from build123d import *

# Parameters (mm, degrees)
SKETCH1_W           = 150
SKETCH1_H           = 150
BOSS_EXTRUDE1_DEPTH = 2.5
CUT_EXTRUDE1_DEPTH  = 5
SKETCH3_R           = 1.55
CUT_EXTRUDE2_DEPTH  = 5
CUT_EXTRUDE3_DEPTH  = 5


with BuildPart() as part:
    # Sketch1 → Boss-Extrude1 (new body, symmetric)
    with BuildSketch(Plane(origin=(0, 0, 0), x_dir=(1, 0, 0), z_dir=(0, 1, 0))):
        Rectangle(SKETCH1_W, SKETCH1_H)
    extrude(amount=BOSS_EXTRUDE1_DEPTH, both=True)

    # Sketch2 → Cut-Extrude1 (cut)
    with BuildSketch(Plane(origin=(0, 2.5, 0), x_dir=(1, 0, 0), z_dir=(0, 1, 0))):
        Polygon((50.251262658, 75), (75, 75), (75, 50.251262658), align=None)
        Polygon((-75, 75), (-75, 50.251262658), (-50.251262658, 75), align=None)
        Polygon((-50.251262658, -75), (-75, -75), (-75, -50.251262658), align=None)
        Polygon((75, -75), (75, -50.251262658), (50.251262658, -75), align=None)
    extrude(amount=-CUT_EXTRUDE1_DEPTH, mode=Mode.SUBTRACT)

    # Sketch3 → Cut-Extrude2 (cut)
    with BuildSketch(Plane(origin=(0, 2.5, 0), x_dir=(1, 0, 0), z_dir=(0, 1, 0))):
        with Locations((69.343145751, 50.251262658)):
            Circle(SKETCH3_R)
        with Locations((53.786796564, 34.694913472)):
            Circle(SKETCH3_R)
        with Locations((34.694913472, 53.786796564)):
            Circle(SKETCH3_R)
        with Locations((50.251262658, 69.343145751)):
            Circle(SKETCH3_R)
        with Locations((-69.343145751, 50.251262658)):
            Circle(SKETCH3_R)
        with Locations((-53.786796564, 34.694913472)):
            Circle(SKETCH3_R)
        with Locations((-34.694913472, 53.786796564)):
            Circle(SKETCH3_R)
        with Locations((-50.251262658, 69.343145751)):
            Circle(SKETCH3_R)
        with Locations((-53.786796564, -34.694913472)):
            Circle(SKETCH3_R)
        with Locations((-69.343145751, -50.251262658)):
            Circle(SKETCH3_R)
        with Locations((-34.694913472, -53.786796564)):
            Circle(SKETCH3_R)
        with Locations((-50.251262658, -69.343145751)):
            Circle(SKETCH3_R)
        with Locations((69.343145751, -50.251262658)):
            Circle(SKETCH3_R)
        with Locations((53.786796564, -34.694913472)):
            Circle(SKETCH3_R)
        with Locations((34.694913472, -53.786796564)):
            Circle(SKETCH3_R)
        with Locations((50.251262658, -69.343145751)):
            Circle(SKETCH3_R)
    extrude(amount=-CUT_EXTRUDE2_DEPTH, mode=Mode.SUBTRACT)

    # Sketch4 → Cut-Extrude3 (cut)
    with BuildSketch(Plane(origin=(0, 2.5, 0), x_dir=(1, 0, 0), z_dir=(0, 1, 0))):
        with BuildLine():
            Line((24, 26), (54, 26))
            ThreePointArc((54, 26), (55, 25), (54, 24))
            Line((54, 24), (24, 24))
            ThreePointArc((24, 24), (23, 25), (24, 26))
        make_face()
        with BuildLine():
            Line((24, -26), (54, -26))
            ThreePointArc((54, -26), (55, -25), (54, -24))
            Line((54, -24), (24, -24))
            ThreePointArc((24, -24), (23, -25), (24, -26))
        make_face()
        with BuildLine():
            Line((-24, -26), (-54, -26))
            ThreePointArc((-54, -26), (-55, -25), (-54, -24))
            Line((-54, -24), (-24, -24))
            ThreePointArc((-24, -24), (-23, -25), (-24, -26))
        make_face()
        with BuildLine():
            Line((-24, 26), (-54, 26))
            ThreePointArc((-54, 26), (-55, 25), (-54, 24))
            Line((-54, 24), (-24, 24))
            ThreePointArc((-24, 24), (-23, 25), (-24, 26))
        make_face()
    extrude(amount=-CUT_EXTRUDE3_DEPTH, mode=Mode.SUBTRACT)


solid = part.part
Verification items for the finished model (mm, model axes). A direction names the side the tool comes from. Give positions to 0.01 mm unless a question says otherwise; leave off trailing zeros. Order: outer loops, then holes, each group sorted by start corner. A loop starts at its lowest first (then second) coordinate and runs counter-clockwise, first axis right, second up. Notation, with made-up numbers: M 53,19 L 89,19 A23 cw 89,52 Z; hole C 5,50.5 d9. An arc over 180 degrees is marked long. Answer as a JSON object with one key per item and string values. Group by question number.
1) Mould release check, pull along X, two halves, no side actions. Record for faces 1 (the face through (-1, 2.5, -1)), 2 (the face through (39, 0, 24)), 3 (the face through (62.8, 0.04, 62.45)): released by +X, released by -X, zero draft, split by the parting line, or undercut.
2) Cross-section at A-A (x = 40.5). Enter the section's corners in (y, z).
3) Depth check by flat-ended pin: pin 1 Ø1.9 at (x, z) = (-34.69, -53.79) entering from +Y; pin 2 Ø1.5 at (x, y) = (-56.5, 1) entering from +Z. Enter the tip coordinate at first touch or a pass-through.
4) Scan lines: line 1 along Z through (x, y) = (26.5, -1.1); line 2 along Z through (x, y) = (51, 1.25); line 3 along X through (y, z) = (1.35, -53). Record each from-to range of solid material in increasing order. Write a range as [from, to].
5) Cross-section at C-C (y = 1.65). Give the number of separate pieces and of enclosed holes in the cut face, then the cut area to 3 significant figures.
6) Access from +Z, -Z, +X, -X, +Y, -Y to the whole of each face (thin tool, end or side, straight path). Record for faces 4 (the face through (39, 0, -24)), 5 (the face through (-1, 0, 75)).
7) Cross-section at B-B (z = -60). Enter the section's corners in (x, y).
Result sheet:
{
 "1": {"face 1": "zero draft", "face 2": "undercut", "face 3": "released by +X"},
 "2": {"outline": "M -2.5,-75 L 2.5,-75 L 2.5,-26 L -2.5,-26 Z; M -2.5,-24 L 2.5,-24 L 2.5,24 L -2.5,24 Z; M -2.5,26 L 2.5,26 L 2.5,75 L -2.5,75 Z"},
 "3": {"pin 1": "passes through", "pin 2": "stops at z = 69.5"},
 "4": {"line 1": "z = [-75, -26], [-24, 24], [26, 75]", "line 2": "z = [-74.25, -70.7], [-67.99, -26], [-24, 24], [26, 67.99], [70.7, 74.25]", "line 3": "x = [-72.25, -36.03], [-33.36, 33.36], [36.03, 72.25]"},
 "5": {"separate pieces": "1", "enclosed holes": "20", "area": "20,900 mm2"},
 "6": {"face 4": "+Y, -Y", "face 5": "+Z, +X, -X, +Y, -Y"},
 "7": {"outline": "M -65.25,-2.5 L 65.25,-2.5 L 65.25,2.5 L -65.25,2.5 Z"}
}
